The listing builds one solid part. Answer for the finished solid, in the listing's coordinates (mm). Face numbers are marked on the shaded views. A direction names the side the tool comes from. Give positions to 0.01 mm unless a question says otherwise; leave off trailing zeros. Order: outer loops, then holes, each group sorted by start corner. A loop starts at its lowest first (then second) coordinate and runs counter-clockwise, first axis right, second up. Notation, with made-up numbers: (74, -36) - (107, -36) arc R21 cw to (107, -32) - close; hole circle Ø6 at (17.25, -22.5). An arc over 180 degrees is marked (long way). Answer in a Markdown table with one row per item.
Autodesk Inventor part; units mm, degrees
ref_plane "YZ Plane" through (0, 0, 0) normal (1, 0, 0) x (0, 1, 0)
ref_plane "XZ Plane" through (0, 0, 0) normal (0, 1, 0) x (-1, 0, 0)
ref_plane "XY Plane" through (0, 0, 0) normal (0, 0, 1) x (1, 0, 0)
sketch "スケッチ1" plane through (0, 0, 0) normal (0, 0, 1) x (1, 0, 0)
  arc A0 (17.1875, -5) -> (17.1875, 5) centre (0, 0) ccw
  line L0 (17.9, -5) -> (12.6, -5)
  line L1 (12.6, -5) -> (12.6, 5)
  line L2 (12.6, 5) -> (17.9, 5)
  line L3 (17.9, 5) -> (17.9, -5)
  point P0 (12.6, 0)
  dimension "d0" = 17.9
  dimension "d1" = 10
  dimension "d2" = 5.3
extrude "押し出し1" add sketch "スケッチ1" along normal blind 5.5 contours L0 L1 L2 A0
sketch "スケッチ2" plane through (0, 0, 0) normal (0, 0, -1) x (-1, 0, 0)
  line L0 (-12.6, 5) -> (-12.6, -5)
  line L1 (-12.6, -3.7) -> (-17.9, -3.7)
  line L2 (-17.9, -3.7) -> (-17.9, 3.7)
  line L3 (-17.9, 3.7) -> (-12.6, 3.7)
  line L4 (-12.6, 3.7) -> (-12.6, -3.7)
  line L5 (-12.6, 5) -> (-12.6, -5)
  line L6 (-12.6, -5) -> (-17.1875, -5)
  arc A0 (-17.1875, 5) -> (-17.1875, -5) centre (0, 0) ccw
  line L7 (-12.6, -1.85) -> (-17.9, -1.85)
  line L8 (-17.9, -1.85) -> (-17.9, 1.85)
  line L9 (-17.9, 1.85) -> (-12.6, 1.85)
  line L10 (-12.6, 1.85) -> (-12.6, -1.85)
  point P0 (-12.6, 0)
  point P1 (-12.6, 0)
  point P2 (-17.8041, -1.85)
  point P3 (-17.5134, -3.7)
  point P4 (-17.8041, 1.85)
  point P5 (-17.5134, 3.7)
  dimension "d5" = 1.3
  dimension "d6" = 3.7
extrude "押し出し2" cut sketch "スケッチ2" against normal blind 2.5 contours L0 L9 A0 L3 | L0 L1 A0 L7
sketch "スケッチ3" plane through (0, 0, 0) normal (0, 0, -1) x (-1, 0, 0)
  line L0 (-12.6, -3.7) -> (-17.5134, -3.7)
  line L1 (-17.5134, 3.7) -> (-12.6, 3.7)
  line L2 (-13.6, -3.7) -> (-14.1, -3.7)
  line L3 (-14.1, -3.7) -> (-14.1, 3.7)
  line L4 (-14.1, 3.7) -> (-13.6, 3.7)
  line L5 (-13.6, 3.7) -> (-13.6, -3.7)
  line L6 (-12.6, 1.85) -> (-12.6, -1.85)
  point P0 (0, 0)
  dimension "d9" = 0.5
  dimension "d10" = 1
extrude "押し出し3" cut sketch "スケッチ3" against normal through all
sketch "スケッチ4" plane through (0, 0, 5.5) normal (0, 0, 1) x (1, 0, 0)
  line L0 (12.6, -5) -> (17.1875, -5)
  arc A0 (16.1434, -5) -> (16.1434, 5) centre (0, 0) ccw
  line L1 (17.1875, 5) -> (12.6, 5)
  arc A1 (17.1875, -5) -> (17.1875, 5) centre (0, 0) ccw
  dimension "d13" = 1
extrude "押し出し4" cut sketch "スケッチ4" against normal up to surface (3 mm away)
properties part number "555_CapAccessory_2" material "アセタール樹脂、白"
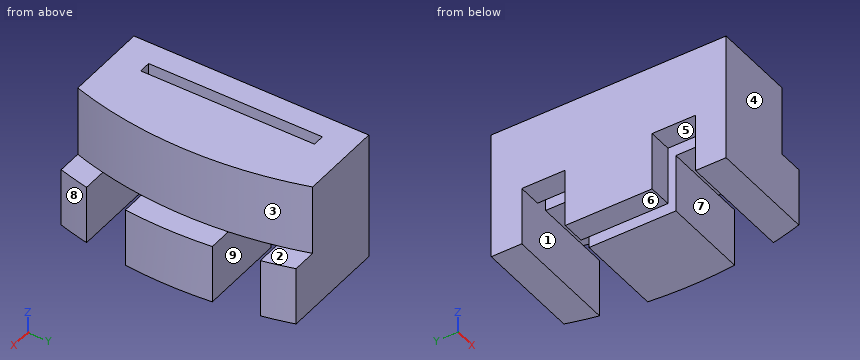
Item 1: Find section B-B on z = 2.75. Write down the section's boundary in (x, y), then the cut area to 3 significant figures.
Answer block:
| item | result |
|---|---|
| outline | (12.6, -5) - (16.14, -5) arc R16.9 ccw to (16.14, 5) - (12.6, 5) - close; hole (13.6, -3.7) - (14.1, -3.7) - (14.1, 3.7) - (13.6, 3.7) - close |
| area | 36.8 mm² |
Item 2: Find section D-D on z = 1.7. Write down the section's boundary in (x, y).
Answer block:
| item | result |
|---|---|
| outline | (12.6, -5) - (17.19, -5) arc R17.9 ccw to (17.51, -3.7) - (12.6, -3.7) - close; (12.6, -1.85) - (13.6, -1.85) - (13.6, 1.85) - (12.6, 1.85) - close; (12.6, 3.7) - (17.51, 3.7) arc R17.9 ccw to (17.19, 5) - (12.6, 5) - close; (14.1, -1.85) - (17.8, -1.85) arc R17.9 ccw to (17.8, 1.85) - (14.1, 1.85) - close |
Item 3: Determine the mould class of the marked faces 6, 7, 8 and 9 for opening direction Y: pulls with the +Y half, pulls with the -Y half, needs draft (parallel to the pull), parting line crosses it, or undercut.
Answer block:
| item | result |
|---|---|
| face 6 | needs draft |
| face 7 | undercut |
| face 8 | pulls with the -Y half |
| face 9 | undercut |
Item 4: Which of the six approach directions +Z, -Z, +X, -X, +Y, -Y give full straight-line access (tool end or side, diameter ignored) to the marked faces 1, 2, 3, 4 and 5?
Answer block:
| item | result |
|---|---|
| face 1 | -Z |
| face 2 | +Z, +X, +Y |
| face 3 | +Z, +X |
| face 4 | +Z, -Z, +X, -X, -Y |
| face 5 | -Z, +X, -X |
Item 5: Find section A-A on x = 13.85. Write down the section's boundary in (y, z).
Answer block:
| item | result |
|---|---|
| outline | (-5, 0) - (-3.7, 0) - (-3.7, 5.5) - (-5, 5.5) - close; (3.7, 0) - (5, 0) - (5, 5.5) - (3.7, 5.5) - close |
Item 6: Consider line 1 (Y direction, x = 16.3, z = 0.65); line 2 (X direction, y = 0.25, z = 2.85); line 3 (Z direction, x = 15.35, y = 2.75). Determine where each line is inside the solid, lowest interval first.
Answer block:
| item | result |
|---|---|
| line 1 | -5 to -3.7, -1.85 to 1.85, 3.7 to 5 |
| line 2 | 12.6 to 13.6, 14.1 to 16.9 |
| line 3 | 2.5 to 5.5 |
Item 7: Each of these flat-tipped pins is pushed along its axis until it touches: P1, Ø0.6, axis at x = 15, y = 2.5, coming from the -Z side; P2, Ø0.6, axis at x = 17.5, y = 0.5, coming from the +Z side. Where does it stop, or does it pass through?
Answer block:
| item | result |
|---|---|
| P1 | z = 2.5 |
| P2 | z = 2.5 |
Item 8: Find section C-C on y = -1.25. Write down the section's boundary in (x, z).
Answer block:
| item | result |
|---|---|
| outline | (12.6, 0) - (13.6, 0) - (13.6, 5.5) - (12.6, 5.5) - close; (14.1, 0) - (17.86, 0) - (17.86, 2.5) - (16.85, 2.5) - (16.85, 5.5) - (14.1, 5.5) - close |
